CAD build for the part. Positions are in the model's coordinates, mm. Face numbers are marked on the shaded views. Coordinates: 2 decimals unless noted, no trailing zeros. Loops run counter-clockwise (first coordinate to the right, second up) from the corner with the lowest first, then second, coordinate; pieces in that order, holes last. Notation, with made-up numbers: (-21.75, -19.75) -> (-2.75, -19.75) arc R13 ccw to (-2.75, -10.75) -> close; hole circle Ø7 at (35, 8). An arc over 180 degrees is marked (long way). Write item = value, one per line. Start each with the question number.
(1) Drill centre lines: line 1 (Y direction, x = -90, z = -3.3); line 2 (X direction, y = 2, z = -0.5); line 3 (Y direction, x = -33, z = -0.95). Where is each one in solid material? Low to high. Write a range as from..to.
(2) Band-saw the part on B-B (x = 3.5). Write the cut outline in (y, z).
(3) Band-saw the part on C-C (x = -63.5). Count the separate pieces of the cut face and the enclosed holes in it, and give its area (3 significant figures).
(4) Band-saw the part on A-A (z = -4.1). Write the cut outline in (x, y).
(5) Pull direction X, two halves, no side cores. Call the marked faces 1 and 2: +X half, -X half, draft (parallel to the pull), parting line (faces both ways), or undercut.
(6) Flat gauge pins, fed straight in: P1, Ø1, axis at y = -13.5, z = -2.5, coming from the +X side; P2, Ø6, axis at x = -26.5, y = 31.5, coming from the -Z side. Where does each tip first touch, or does it go through?
Solid Edge part; units mm, degrees
sketch "Sketch1" plane through (0, 0, 0) normal (0, 0, 1) x (1, 0, 0)
  line L0 (-97.5, -43.5) -> (-97.5, 44)
  arc A0 (-97.5, 44) -> (-90, 51.5) centre (-90, 44) cw
  line L1 (-90, 51.5) -> (90, 51.5)
  arc A1 (90, 51.5) -> (97.5, 44) centre (90, 44) cw
  line L2 (97.5, 44) -> (97.5, -43.5)
  line L3 (97.5, -43.5) -> (-97.5, -43.5)
extrude "Protrusion1" add sketch "Sketch1" against normal blind 1
sketch "Sketch2" plane through (0, 4, 0) normal (0, 0, 1) x (1, 0, 0)
  line L0 (41.76, -27.84) -> (41.76, 27.84)
  line L1 (41.76, 27.84) -> (-41.76, 27.84)
  line L2 (-41.76, 27.84) -> (-41.76, -27.84)
  line L3 (-41.76, -27.84) -> (41.76, -27.84)
extrude "Cutout1" cut sketch "Sketch2" against normal up to vertex (1 mm away)
sketch "Sketch3" plane through (0, 4, -1) normal (0, 0, -1) x (-1, 0, 0)
  circle A0 centre (90, 40) radius 4.7
  circle A1 centre (90, 40) radius 1.7
  circle A2 centre (-90, 40) radius 4.7
  circle A3 centre (-90, 40) radius 1.7
  circle A4 centre (-90, -40) radius 4.7
  circle A5 centre (-90, -40) radius 1.7
  circle A6 centre (90, -40) radius 4.7
  circle A7 centre (90, -40) radius 1.7
extrude "ExtrudedProtrusion_2" add sketch "Sketch3" along normal blind 4
sketch "Sketch4" plane through (0, 4, -1) normal (0, 0, -1) x (-1, 0, 0)
  circle A0 centre (-90, 40) radius 1.7
  circle A1 centre (-90, -40) radius 1.7
  circle A2 centre (90, -40) radius 1.7
  circle A3 centre (90, 40) radius 1.7
extrude "Cutout2" cut sketch "Sketch4" against normal up to vertex (1 mm away)
chamfer "Chamfer_1" distance 2 angle 45 4 edges at (-88.3, 44, 0) (91.7, 44, 0) (91.7, -36, 0) (-88.3, -36, 0)
sketch "Sketch5" plane through (0, 4, 0) normal (0, 0, 1) x (1, 0, 0)
  line L0 (-59.63, 23.5) -> (-79.63, 23.5)
  line L1 (-79.63, 23.5) -> (-79.63, 22.5)
  line L2 (-79.63, 22.5) -> (-59.63, 22.5)
  line L3 (-59.63, 22.5) -> (-59.63, 23.5)
  line L4 (-79.63, 19.5) -> (-59.63, 19.5)
  line L5 (-59.63, 19.5) -> (-59.63, 20.5)
  line L6 (-59.63, 20.5) -> (-79.63, 20.5)
  line L7 (-79.63, 20.5) -> (-79.63, 19.5)
  line L8 (-79.63, 16.5) -> (-59.63, 16.5)
  line L9 (-59.63, 16.5) -> (-59.63, 17.5)
  line L10 (-59.63, 17.5) -> (-79.63, 17.5)
  line L11 (-79.63, 17.5) -> (-79.63, 16.5)
  line L12 (-59.63, 11.5) -> (-79.63, 11.5)
  line L13 (-79.63, 11.5) -> (-79.63, 10.5)
  line L14 (-79.63, 10.5) -> (-59.63, 10.5)
  line L15 (-59.63, 10.5) -> (-59.63, 11.5)
  line L16 (-79.63, 13.5) -> (-59.63, 13.5)
  line L17 (-59.63, 13.5) -> (-59.63, 14.5)
  line L18 (-59.63, 14.5) -> (-79.63, 14.5)
  line L19 (-79.63, 14.5) -> (-79.63, 13.5)
  line L20 (-79.63, 7.5) -> (-59.63, 7.5)
  line L21 (-59.63, 7.5) -> (-59.63, 8.5)
  line L22 (-59.63, 8.5) -> (-79.63, 8.5)
  line L23 (-79.63, 8.5) -> (-79.63, 7.5)
  line L24 (-59.63, 5.5) -> (-79.63, 5.5)
  line L25 (-79.63, 5.5) -> (-79.63, 4.5)
  line L26 (-79.63, 4.5) -> (-59.63, 4.5)
  line L27 (-59.63, 4.5) -> (-59.63, 5.5)
  line L28 (-79.63, 1.5) -> (-59.63, 1.5)
  line L29 (-59.63, 1.5) -> (-59.63, 2.5)
  line L30 (-59.63, 2.5) -> (-79.63, 2.5)
  line L31 (-79.63, 2.5) -> (-79.63, 1.5)
  line L32 (-79.63, -2.5) -> (-59.63, -2.5)
  line L33 (-59.63, -2.5) -> (-59.63, -1.5)
  line L34 (-59.63, -1.5) -> (-79.63, -1.5)
  line L35 (-79.63, -1.5) -> (-79.63, -2.5)
  line L36 (-79.63, -5.5) -> (-59.63, -5.5)
  line L37 (-59.63, -5.5) -> (-59.63, -4.5)
  line L38 (-59.63, -4.5) -> (-79.63, -4.5)
  line L39 (-79.63, -4.5) -> (-79.63, -5.5)
  line L40 (-79.63, -8.5) -> (-59.63, -8.5)
  line L41 (-59.63, -8.5) -> (-59.63, -7.5)
  line L42 (-59.63, -7.5) -> (-79.63, -7.5)
  line L43 (-79.63, -7.5) -> (-79.63, -8.5)
  line L44 (-79.63, -11.5) -> (-59.63, -11.5)
  line L45 (-59.63, -11.5) -> (-59.63, -10.5)
  line L46 (-59.63, -10.5) -> (-79.63, -10.5)
  line L47 (-79.63, -10.5) -> (-79.63, -11.5)
  line L48 (-79.63, -14.5) -> (-59.63, -14.5)
  line L49 (-59.63, -14.5) -> (-59.63, -13.5)
  line L50 (-59.63, -13.5) -> (-79.63, -13.5)
  line L51 (-79.63, -13.5) -> (-79.63, -14.5)
  line L52 (-59.63, -16.5) -> (-79.63, -16.5)
  line L53 (-79.63, -16.5) -> (-79.63, -17.5)
  line L54 (-79.63, -17.5) -> (-59.63, -17.5)
  line L55 (-59.63, -17.5) -> (-59.63, -16.5)
  line L56 (-79.63, -20.5) -> (-59.63, -20.5)
  line L57 (-59.63, -20.5) -> (-59.63, -19.5)
  line L58 (-59.63, -19.5) -> (-79.63, -19.5)
  line L59 (-79.63, -19.5) -> (-79.63, -20.5)
  line L60 (-59.63, -22.5) -> (-79.63, -22.5)
  line L61 (-79.63, -22.5) -> (-79.63, -23.5)
  line L62 (-79.63, -23.5) -> (-59.63, -23.5)
  line L63 (-59.63, -23.5) -> (-59.63, -22.5)
extrude "Cutout3" cut sketch "Sketch5" against normal up to vertex (1 mm away)
properties material "Polycarbonate"
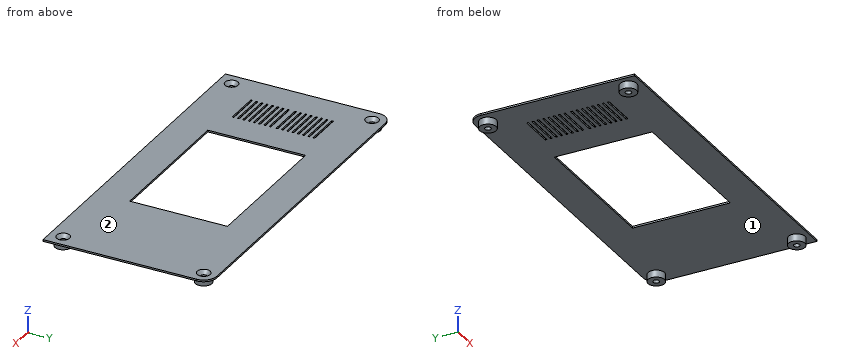
Findings below:
q1.line_1 = -40.7..-37.7, -34.3..-31.3, 39.3..42.3, 45.7..48.7
q1.line_2 = -97.5..-79.63, -59.63..-41.76, 41.76..97.5
q1.line_3 = -43.5..-23.84, 31.84..51.5
q2.outline = (-43.5, -1) -> (-23.84, -1) -> (-23.84, 0) -> (-43.5, 0) -> close; (31.84, -1) -> (51.5, -1) -> (51.5, 0) -> (31.84, 0) -> close
q3.separate_pieces = 17
q3.enclosed_holes = 0
q3.area = 79.0 mm²
q4.outline = circle Ø9.4 at (-90, -36); circle Ø9.4 at (-90, 44); circle Ø9.4 at (90, -36); circle Ø9.4 at (90, 44); hole circle Ø3.4 at (-90, -36); hole circle Ø3.4 at (-90, 44); hole circle Ø3.4 at (90, -36); hole circle Ø3.4 at (90, 44)
q5.face_1 = undercut
q5.face_2 = draft
q6.P1 = through
q6.P2 = -1
